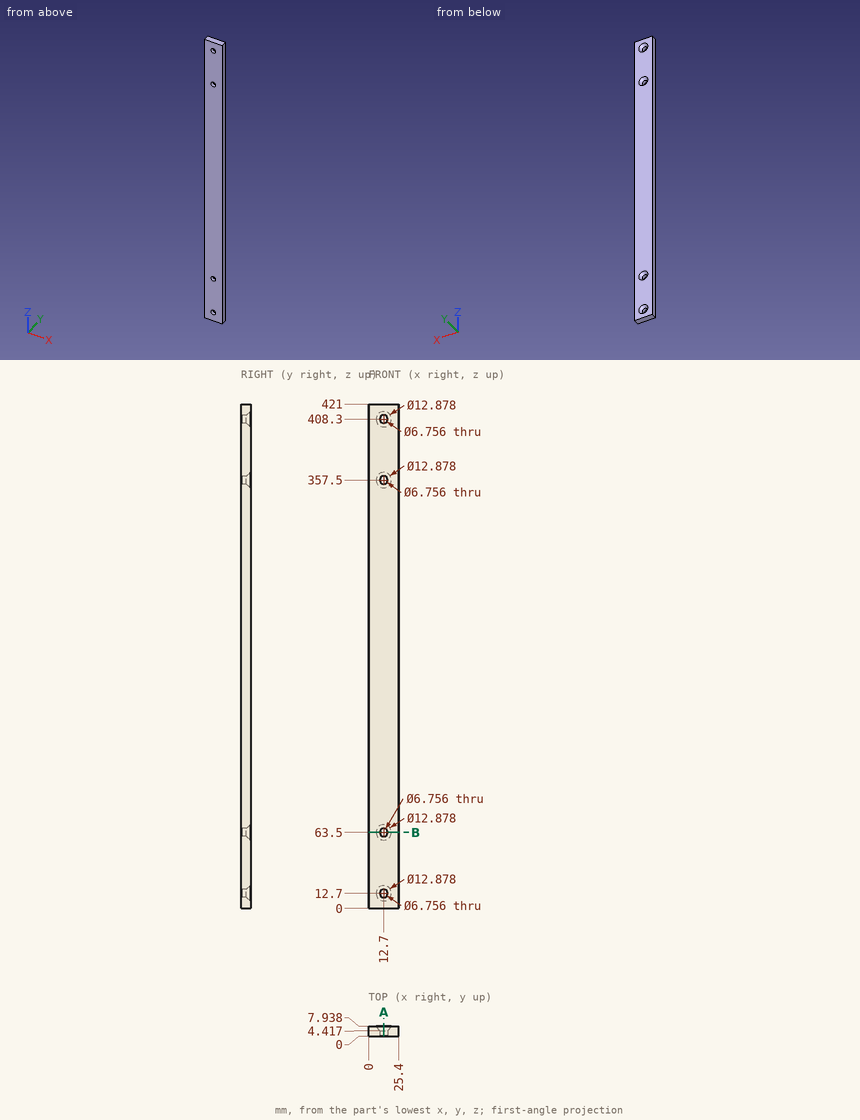
Verification items for this drawing (mm, ordinates from the low corner). Coordinates: 2 decimals unless noted, no trailing zeros. Order: outer loops, then holes, each group sorted by start corner. A loop starts at its lowest first (then second) coordinate and runs counter-clockwise, first axis right, second up. Notation, with made-up numbers: M 78.25,-29 L 95.25,-29 A31 cw 95.25,-2 Z; hole C 65.5,30.5 d7. An arc over 180 degrees is marked long. One line per item, written item: value. Start each with the question number.
Item 1: Depth check by flat-ended pin: P1, Ø5.5, axis at x = 12.7, z = 63.5, coming from the +Y side; P2, Ø9, axis at x = 12.7, z = 12.7, coming from the +Y side (1 decimal). Enter the tip coordinate at first touch or a pass-through.
Item 2: Thickness scan on probe 1 along Z at (x, y) = (12.7, 0.9); probe 2 along X at (y, z) = (1.65, 12.7); probe 3 along Z at (x, y) = (10.25, 4.25) (1 decimal). Record the ranges inside material, lowest first.
Item 3: Sectioned sample at A-A on x = 12.7. Record the cut outline in (y, z).
Item 4: Sectioned sample at B-B on z = 63.5. Record the cut outline in (x, y), then the cut area to 3 significant figures.
Calculated:
1. P1: through
1. P2: y = 5.7
2. probe 1: 0 to 9.32, 16.08 to 60.12, 66.88 to 354.12, 360.88 to 404.92, 411.68 to 421
2. probe 2: 0 to 9.32, 16.08 to 25.4
2. probe 3: 0 to 10.4, 15 to 61.2, 65.8 to 355.2, 359.8 to 406, 410.6 to 421
3. outline: M 0,0 L 7.94,0 L 7.94,6.26 L 4.42,9.32 L 0,9.32 Z; M 0,16.08 L 4.42,16.08 L 7.94,19.14 L 7.94,57.06 L 4.42,60.12 L 0,60.12 Z; M 0,66.88 L 4.42,66.88 L 7.94,69.94 L 7.94,351.06 L 4.42,354.12 L 0,354.12 Z; M 0,360.88 L 4.42,360.88 L 7.94,363.94 L 7.94,401.86 L 4.42,404.92 L 0,404.92 Z; M 0,411.68 L 4.42,411.68 L 7.94,414.74 L 7.94,421 L 0,421 Z
4. outline: M 0,0 L 9.32,0 L 9.32,4.42 L 6.26,7.94 L 0,7.94 Z; M 16.08,0 L 25.4,0 L 25.4,7.94 L 19.14,7.94 L 16.08,4.42 Z
4. area: 137 mm^2
